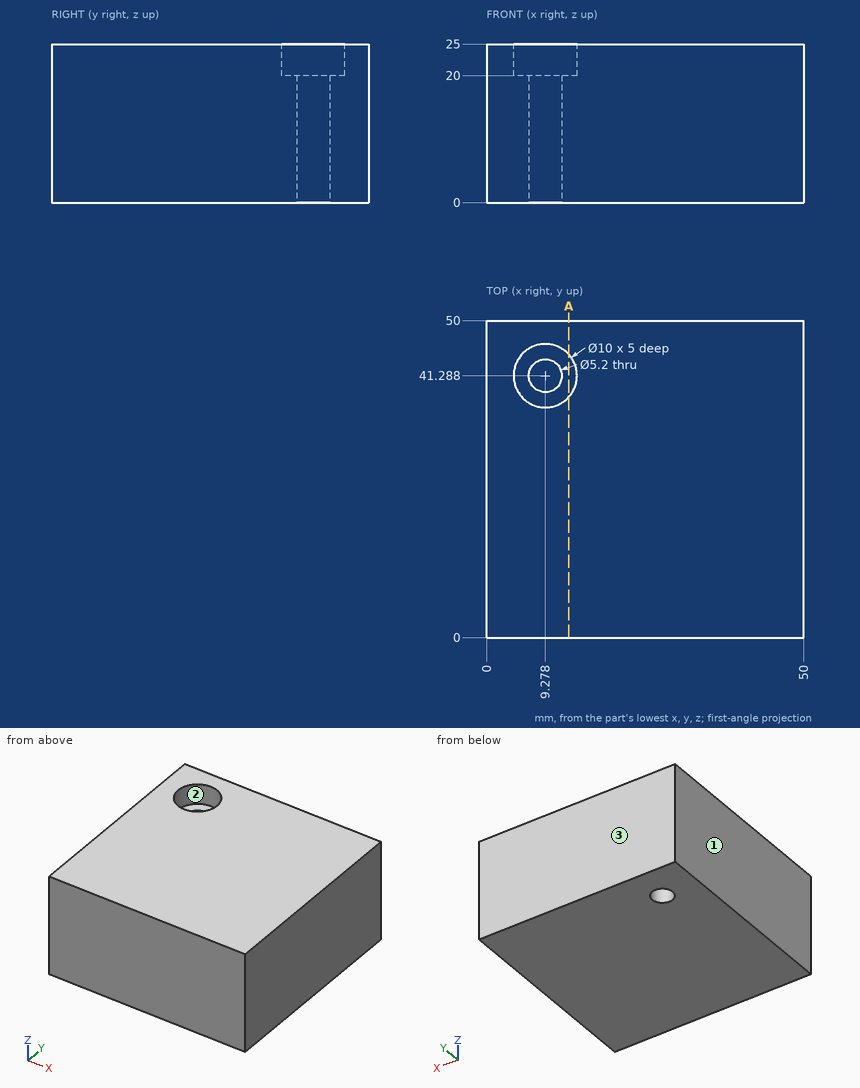
Can you work these out from the drawing? Everything is in mm from the part's minimum corner. Give positions to 0.01 mm unless a question says otherwise; leave off trailing zeros. Order: outer loops, then holes, each group sorted by start corner. A loop starts at its lowest first (then second) coordinate and runs counter-clockwise, first axis right, second up. Notation, with made-up numbers: M 10.5,62.25 L 17.5,62.25 A18 ccw 17.5,81.25 Z; hole C 17.25,40 d3. An arc over 180 degrees is marked long. Use a Markdown table: item, result. Add a question column.
1. I need wall thicknesses on probe 1 along Y at (x, z) = (9, 24); probe 2 along Y at (x, z) = (9.5, 13.25). Which ranges of each line are inside material? Lowest first, please. Write a range as from..to.
2. For pin 1 Ø7 at (x, y) = (9.28, 41.29) entering from +Z, with a flat end and sliding along its axis, tell me the tip position at first contact or that it passes through.
3. If we mould it in two halves opening along Y, with no side actions, what happens to the marked faces 1, 2 and 3? For each: +Y half, -Y half, draft (parallel to the pull), parting line (faces both ways), or undercut.
4. Suppose I cut it at A-A (x = 13). List the corners of the cut face in (y, z) for me.
Results list:
| question | item | result |
|---|---|---|
| 1 | probe 1 | y = 0..36.3, 46.28..50 |
| 1 | probe 2 | y = 0..38.7, 43.88..50 |
| 2 | pin 1 | stops at z = 20 |
| 3 | face 1 | draft |
| 3 | face 2 | undercut |
| 3 | face 3 | +Y half |
| 4 | outline | M 0,0 L 50,0 L 50,25 L 44.63,25 L 44.63,20 L 37.95,20 L 37.95,25 L 0,25 Z |
